from build123d import *

# Parameters (mm, degrees)
SKETCH_1_R             = 10
SM_BASE_FLANGE_1_DEPTH = 4


# Sheet-metal steps are written as plain solids
with BuildPart() as part:
    # Sketch 1 → Базовая кромка1 (new body)
    with BuildSketch(Plane.XY):
        Polygon((-25, 16), (-25, -65), (-18, -65), (-18, -72), (-11, -72), (-11, -79), (11, -79), (11, -72), (18, -72), (18, -65), (25, -65), (25, 16), (18, 16), (18, 23), (11, 23), (11, 30), (-11, 30), (-11, 23), (-18, 23), (-18, 16), align=None)
        Circle(SKETCH_1_R, mode=Mode.SUBTRACT)
        with Locations((0, -49)):
            Circle(SKETCH_1_R, mode=Mode.SUBTRACT)
    extrude(amount=-SM_BASE_FLANGE_1_DEPTH)


solid = part.part
Design review of the part built by this model. Coordinates are the model's own, in mm. A direction names the side the tool comes from. Round coordinates to 2 decimals unless told otherwise and drop trailing zeros. Write each loop counter-clockwise with the first axis right and the second up, starting at its lowest first coordinate (ties: lowest second). Pieces come first, ordered by that corner, then holes.
Item 1: Consider section C-C on z = -1.95. Give the boundary of the cut face in (x, y).
Item 2: For faces 1 (the flat face through (-11, 27, -2)), 2 (the flat face through (21, -65, -2)), 3 (the flat face through (11, 26, -2)), 4 (the flat face through (-15, -72, -2)), list the 3-axis set-ups (+Z, -Z, +X, -X, +Y, -Y) from which the entire face can be reached by the end or side of a thin tool; tool diameter is ignored.
Item 3: Wall thickness on L1, parallel to Y at x = 0, z = -2.15; L2, parallel to Y at x = 2.5, z = -0.2; L3, parallel to Y at x = -12, z = -1.45: over which ranges is each line inside the solid? List them lowest first.
Item 4: Consider section A-A on x = 0. Give the boundary of the cut face in (y, z).
Item 5: Draft analysis for pull direction X (two halves, no side actions). For faces 5 (the flat face through (-21, 16, -2)), 6 (the flat face through (-18, 20, -2)), 7 (the cylindrical face through (-2.17, -58.76, -1.97)), state which applies: released by +X, released by -X, zero draft, split by the parting line, or undercut.
Item 6: Consider section B-B on y = -49. Give the boundary of the cut face in (x, z).
Item 7: For pin 1 Ø1.2 at (x, z) = (-14, -2.5) entering from -Y; pin 2 Ø1.2 at (x, z) = (-13, -1) entering from +Y; pin 3 Ø2 at (y, z) = (-67.5, -3) entering from +X, all flat-tipped, find the tip position at first contact; note any pin that passes through.
Check values:
1. outline: (-25, -65) - (-18, -65) - (-18, -72) - (-11, -72) - (-11, -79) - (11, -79) - (11, -72) - (18, -72) - (18, -65) - (25, -65) - (25, 16) - (18, 16) - (18, 23) - (11, 23) - (11, 30) - (-11, 30) - (-11, 23) - (-18, 23) - (-18, 16) - (-25, 16) - close; hole circle Ø20 at (0, -49); hole circle Ø20 at (0, 0)
2. face 1: +Z, -Z, -X, +Y
2. face 2: +Z, -Z, +X, -Y
2. face 3: +Z, -Z, +X, +Y
2. face 4: +Z, -Z, -X, -Y
3. L1: y = -79 to -59, -39 to -10, 10 to 30
3. L2: y = -79 to -58.68, -39.32 to -9.68, 9.68 to 30
3. L3: y = -72 to 23
4. outline: (-79, -4) - (-59, -4) - (-59, 0) - (-79, 0) - close; (-39, -4) - (-10, -4) - (-10, 0) - (-39, 0) - close; (10, -4) - (30, -4) - (30, 0) - (10, 0) - close
5. face 5: zero draft
5. face 6: released by -X
5. face 7: undercut
6. outline: (-25, -4) - (-10, -4) - (-10, 0) - (-25, 0) - close; (10, -4) - (25, -4) - (25, 0) - (10, 0) - close
7. pin 1: stops at y = -72
7. pin 2: stops at y = 23
7. pin 3: stops at x = 18
